Read the model definition and answer for the solid it produces. Units are mm, in the model's axes. Face numbers are marked on the shaded views. A direction names the side the tool comes from. Coordinates: 2 decimals unless noted, no trailing zeros. Loops run counter-clockwise (first coordinate to the right, second up) from the corner with the lowest first, then second, coordinate; pieces in that order, holes last. Notation, with made-up numbers: M 10,64.25 L 42,64.25 A20 cw 42,71.25 Z; hole C 13,-4.5 d4. An arc over 180 degrees is marked long. One line per item, written item: value. Start each with the question number.
1. Determine the mould class of the marked faces 4 and 5 for opening direction Z: +Z half, -Z half, draft (parallel to the pull), parting line (faces both ways), or undercut.
2. Flat-ended cylindrical pins translate along their axes: pin 1 (1.2 mm diameter, centred on x = 2.5, z = -19, fed in from -Y); pin 2 (1 mm diameter, centred on x = 0.5, y = 1, fed in from +Z). Find the tip coordinate at first contact, or state that the pin passes through.
3. The part is cut by section B-B (z = -42). Write down the section's boundary in (x, y), then the cut area to 3 significant figures.
4. The part is cut by section D-D (y = -2.75). Write down the section's boundary in (x, z).
5. Consider probe 1 along Y at (x, z) = (2.65, 0); probe 2 along Z at (x, y) = (1.25, 1); probe 3 along Z at (x, y) = (1.15, -0.5). Determine where each line is inside the solid, lowest interval first.
6. The part is cut by section A-A (y = 0). Write down the section's boundary in (x, z), then the cut area to 3 significant figures.
7. For the marked faces 1, 2 and 3, determine the directions among +Z, -Z, +X, -X, +Y, -Y from which every point of the face is accessible in a straight line to the end or side of a thin tool.
8. The part is cut by section C-C (x = 3.2). Write down the section's boundary in (y, z).
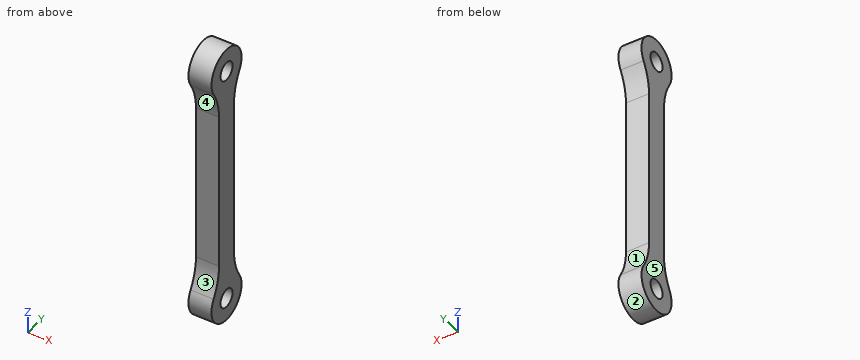
```python
from build123d import *

# Parameters (mm, degrees)
SKETCH1_R           = 1.6
BOSS_EXTRUDE1_DEPTH = 4
FILLET1_R           = 10


with BuildPart() as part:
    # Sketch1 → Boss-Extrude1 (new body)
    with BuildSketch(Plane(origin=(0, 0, 0), x_dir=(0, 0, -1), z_dir=(1, 0, 0))):
        with BuildLine():
            Line((21, 2), (38.535898385, 2))
            ThreePointArc((38.535898385, 2), (46, 0), (38.535898385, -2))
            Line((38.535898385, -2), (21, -2))
            Line((21, -2), (3.464101615, -2))
            ThreePointArc((3.464101615, -2), (-4, 0), (3.464101615, 2))
            Line((3.464101615, 2), (21, 2))
        make_face()
        Circle(SKETCH1_R, mode=Mode.SUBTRACT)
        with Locations((42, 0)):
            Circle(SKETCH1_R, mode=Mode.SUBTRACT)
    extrude(amount=BOSS_EXTRUDE1_DEPTH)

    # Fillet1
    fillet1_edges = [part.edges().sort_by_distance(p)[0] for p in [
        (2, 2, -38.535898385),
        (2, -2, -38.535898385),
        (2, -2, -3.464101615),
        (2, 2, -3.464101615),
    ]]
    fillet(fillet1_edges, radius=FILLET1_R)


solid = part.part
```
Answer block:
1. face 4: undercut
1. face 5: draft
2. pin 1: stops at y = -2
2. pin 2: stops at z = 3.97
3. outline: M 0,-4 L 4,-4 L 4,-1.6 L 0,-1.6 Z; M 0,1.6 L 4,1.6 L 4,4 L 0,4 Z
3. area: 19.2 mm2
4. outline: M 0,-44.9 L 4,-44.9 L 4,-38.59 L 0,-38.59 Z; M 0,-3.41 L 4,-3.41 L 4,2.9 L 0,2.9 Z
5. probe 1: y = -4 to -1.6, 1.6 to 4
5. probe 2: z = -45.87 to -43.25, -40.75 to -1.25, 1.25 to 3.87
5. probe 3: z = -45.97 to -43.52, -40.48 to -1.52, 1.52 to 3.97
6. outline: M 0,-46 L 4,-46 L 4,-43.6 L 0,-43.6 Z; M 0,-40.4 L 4,-40.4 L 4,-1.6 L 0,-1.6 Z; M 0,1.6 L 4,1.6 L 4,4 L 0,4 Z
6. area: 174 mm2
7. face 1: +X, -X, +Y
7. face 2: +X, -X
7. face 3: +X, -X, -Y
8. outline: M -3.43,-39.94 A4 ccw long 3.43,-39.94 A10 cw 2,-34.79 L 2,-7.21 A10 cw 3.43,-2.06 A4 ccw long -3.43,-2.06 A10 cw -2,-7.21 L -2,-34.79 A10 cw Z; hole C 0,-42 d3.2; hole C 0,0 d3.2
